The model under review builds one solid part; all positions refer to its coordinate system, in mm. A direction names the side the tool comes from. Round coordinates to 2 decimals unless told otherwise and drop trailing zeros. Order: outer loops, then holes, each group sorted by start corner. A loop starts at its lowest first (then second) coordinate and runs counter-clockwise, first axis right, second up. Notation, with made-up numbers: M -12.5,62 L 32.5,62 A13 ccw 32.5,87 Z; hole C 79,-25 d4. An arc over 180 degrees is marked long. Use a Markdown table: item, result. Add a question column.
1. Insertion check: P1, Ø12, axis at x = 7, z = 6, coming from the +Y side; P2, Ø8, axis at x = 9.5, y = 94.5, coming from the -Z side; P3, Ø5, axis at y = 84.5, z = -6.5, coming from the +X side; P4, Ø4, axis at x = 5.5, z = -13, coming from the -Y side. Each pin has a flat end and moves straight along its axis. Give the tip position at first contact, or say it passes through.
2. Consider section B-B on z = 15. State the section outline as (x, y) points, then the cut area to 3 significant figures.
3. Consider section A-A on x = -10. State the section outline as (y, z) points, then the cut area to 3 significant figures.
4. For faces 1 (the flat face through (-18.5, 148, 0)), 2 (the flat face through (0, 5, -18.3)), 3 (the flat face through (-4, 6.5, 4)), 4 (the flat face through (-1.9, 151, 0)), list the 3-axis set-ups (+Z, -Z, +X, -X, +Y, -Y) from which the entire face can be reached by the end or side of a thin tool; tool diameter is ignored.
5. To check wall thickness, follow probe 1 along Y at (x, z) = (-17, 1); probe 2 along Z at (x, y) = (1, 22.5); probe 3 along X at (y, z) = (7.5, 3). State the ranges of each line that lie inside material, in increasing order.
6. The part is to be moulded in two halves that separate along Y. For faces 5 (the cylindrical face through (0, 13.7, -2.8)), 6 (the flat face through (3, 153, 0)), 7 (the flat face through (0, 10, -18.3)), 8 (the cylindrical face through (-4.88, 7.49, -1.08)), say which applies: +Y half, -Y half, draft (parallel to the pull), parting line (faces both ways), or undercut.
7. Consider section C-C on y = 48. State the section outline as (x, z) points, then the cut area to 3 significant figures.
from build123d import *

# Parameters (mm, degrees)
BOSS_EXTRUDE1_DEPTH     = 6.5
SKETCH2_R               = 20
BOSS_EXTRUDE2_DEPTH     = 2.5
CUT_EXTRUDE1_DEPTH      = 8
SKETCH4_W               = 3
SKETCH4_H               = 3
CUT_EXTRUDE2_DEPTH      = 10
SKETCH5_R               = 5
BOSS_EXTRUDE3_DEPTH     = 140
CUT_EXTRUDE3_DEPTH      = 10
MIRROR5_COPY_1_SKETCH_R = 20
MIRROR5_COPY_1_DEPTH    = 2.5
MIRROR5_COPY_2_SKETCH_W = 3
MIRROR5_COPY_2_SKETCH_H = 3
MIRROR5_COPY_2_DEPTH    = 10


with BuildPart() as part:
    # Sketch1 → Boss-Extrude1 (new body)
    with BuildSketch(Plane(origin=(0, 0, 0), x_dir=(1, 0, 0), z_dir=(0, 1, 0))):
        with BuildLine():
            ThreePointArc((-1.9, -2.05669638), (-2.8, 0), (-1.9, 2.05669638))
            Line((-1.9, 2.05669638), (-1.9, 5.532856405))
            ThreePointArc((-1.9, 5.532856405), (-5.85, 0), (-1.9, -5.532856405))
            Line((-1.9, -5.532856405), (-1.9, -2.05669638))
        make_face()
        with BuildLine():
            ThreePointArc((-1.9, 2.05669638), (0, 2.8), (1.9, 2.05669638))
            Line((1.9, 2.05669638), (1.9, 5.532856405))
            ThreePointArc((1.9, 5.532856405), (0, 5.85), (-1.9, 5.532856405))
            Line((-1.9, 5.532856405), (-1.9, 2.05669638))
        make_face()
        with BuildLine():
            Line((1.9, 5.532856405), (1.9, 2.05669638))
            ThreePointArc((1.9, 2.05669638), (2.565151068, 1.122497216), (2.8, 0))
            ThreePointArc((2.8, 0), (2.565151068, -1.122497216), (1.9, -2.05669638))
            Line((1.9, -2.05669638), (1.9, -5.532856405))
            ThreePointArc((1.9, -5.532856405), (4.761171074, -3.399080758), (5.85, 0))
            ThreePointArc((5.85, 0), (4.761171074, 3.399080758), (1.9, 5.532856405))
        make_face()
        with BuildLine():
            Line((1.9, -5.532856405), (1.9, -2.05669638))
            ThreePointArc((1.9, -2.05669638), (0, -2.8), (-1.9, -2.05669638))
            Line((-1.9, -2.05669638), (-1.9, -5.532856405))
            ThreePointArc((-1.9, -5.532856405), (0, -5.85), (1.9, -5.532856405))
        make_face()
        with BuildLine():
            Line((-1.9, -2.05669638), (-1.9, 2.05669638))
            ThreePointArc((-1.9, 2.05669638), (-2.8, 0), (-1.9, -2.05669638))
        make_face()
        with BuildLine():
            ThreePointArc((2.8, 0), (2.565151068, 1.122497216), (1.9, 2.05669638))
            Line((1.9, 2.05669638), (1.9, -2.05669638))
            ThreePointArc((1.9, -2.05669638), (2.565151068, -1.122497216), (2.8, 0))
        make_face()
    boss_extrude1 = extrude(amount=BOSS_EXTRUDE1_DEPTH)

    # Sketch2 → Boss-Extrude2 (add)
    with BuildSketch(Plane(origin=(0, 6.5, 0), x_dir=(1, 0, 0), z_dir=(0, 1, 0))):
        with Locations(Location((0, 0, 0), (0, 0, 270))):
            Circle(SKETCH2_R)
    boss_extrude2 = extrude(amount=-BOSS_EXTRUDE2_DEPTH)

    # Sketch3 → Cut-Extrude1 (cut)
    with BuildSketch(Plane.XZ.offset(-4)):
        with BuildLine():
            Line((-1.9, 2.05669638), (-1.9, -2.05669638))
            ThreePointArc((-1.9, -2.05669638), (0, -2.8), (1.9, -2.05669638))
            Line((1.9, -2.05669638), (1.9, 2.05669638))
            ThreePointArc((1.9, 2.05669638), (0, 2.8), (-1.9, 2.05669638))
        make_face()
    extrude(amount=-CUT_EXTRUDE1_DEPTH, mode=Mode.SUBTRACT)

    # Sketch4 → Cut-Extrude2 (cut)
    with BuildSketch(Plane(origin=(0, 6.5, 0), x_dir=(1, 0, 0), z_dir=(0, 1, 0))):
        with Locations((0, 19.8)):
            Rectangle(SKETCH4_W, SKETCH4_H)
        with Locations((20, 0)):
            Rectangle(SKETCH4_W, SKETCH4_H)
        with Locations((0, -20)):
            Rectangle(SKETCH4_W, SKETCH4_H)
        with Locations((-20, 0)):
            Rectangle(SKETCH4_W, SKETCH4_H)
    cut_extrude2 = extrude(amount=-CUT_EXTRUDE2_DEPTH, mode=Mode.SUBTRACT)

    # Sketch5 → Boss-Extrude3 (add)
    with BuildSketch(Plane(origin=(0, 6.5, 0), x_dir=(1, 0, 0), z_dir=(0, 1, 0))):
        with Locations(Location((0, 0, 0), (0, 0, 270))):
            Circle(SKETCH5_R)
    extrude(amount=BOSS_EXTRUDE3_DEPTH)

    # Mirror1: Boss-Extrude2, Cut-Extrude2 across plane
    add(boss_extrude2.mirror(Plane.ZX.offset(76.5)))
    add(cut_extrude2.mirror(Plane.ZX.offset(76.5)), mode=Mode.SUBTRACT)

    # Mirror2: Boss-Extrude1 across plane
    add(boss_extrude1.mirror(Plane.ZX.offset(76.5)))

    # Sketch6 → Cut-Extrude3 (cut)
    with BuildSketch(Plane.XZ.offset(-6.5)):
        with BuildLine():
            Line((-1.9, 2.05669638), (-1.9, -2.05669638))
            ThreePointArc((-1.9, -2.05669638), (0, -2.8), (1.9, -2.05669638))
            Line((1.9, -2.05669638), (1.9, 2.05669638))
            ThreePointArc((1.9, 2.05669638), (0, 2.8), (-1.9, 2.05669638))
        make_face()
    extrude(amount=-CUT_EXTRUDE3_DEPTH, mode=Mode.SUBTRACT)

    # Mirror3: Boss-Extrude2, Cut-Extrude2 across plane
    add(boss_extrude2.mirror(Plane.ZX.offset(7.5)))
    add(cut_extrude2.mirror(Plane.ZX.offset(7.5)), mode=Mode.SUBTRACT)

    # Mirror5 copy 1 sketch → Mirror5 copy 1 (add)
    with BuildSketch(Plane(origin=(0, 144.5, 0), x_dir=(1, 0, 0), z_dir=(0, 1, 0))):
        with Locations(Location((0, 0, 0), (0, 0, 270))):
            Circle(MIRROR5_COPY_1_SKETCH_R)
    extrude(amount=-MIRROR5_COPY_1_DEPTH)

    # Mirror5 copy 2 sketch → Mirror5 copy 2 (cut)
    with BuildSketch(Plane(origin=(0, 144.5, 0), x_dir=(1, 0, 0), z_dir=(0, 1, 0))):
        with Locations((0, 19.8)):
            Rectangle(MIRROR5_COPY_2_SKETCH_W, MIRROR5_COPY_2_SKETCH_H)
        with Locations((20, 0)):
            Rectangle(MIRROR5_COPY_2_SKETCH_W, MIRROR5_COPY_2_SKETCH_H)
        with Locations((0, -20)):
            Rectangle(MIRROR5_COPY_2_SKETCH_W, MIRROR5_COPY_2_SKETCH_H)
        with Locations((-20, 0)):
            Rectangle(MIRROR5_COPY_2_SKETCH_W, MIRROR5_COPY_2_SKETCH_H)
    extrude(amount=-MIRROR5_COPY_2_DEPTH, mode=Mode.SUBTRACT)


solid = part.part
Answer block:
| question | item | result |
|---|---|---|
| 1 | P1 | y = 153 |
| 1 | P2 | through |
| 1 | P3 | x = 3 |
| 1 | P4 | y = 4 |
| 2 | outline | M -13.23,4 L 13.23,4 L 13.23,6.5 L -13.23,6.5 Z; M -13.23,8.5 L 13.23,8.5 L 13.23,11 L -13.23,11 Z; M -13.23,142 L 13.23,142 L 13.23,144.5 L -13.23,144.5 Z; M -13.23,146.5 L 13.23,146.5 L 13.23,149 L -13.23,149 Z |
| 2 | area | 265 mm^2 |
| 3 | outline | M 4,-17.32 L 6.5,-17.32 L 6.5,17.32 L 4,17.32 Z; M 8.5,-17.32 L 11,-17.32 L 11,17.32 L 8.5,17.32 Z; M 142,-17.32 L 144.5,-17.32 L 144.5,17.32 L 142,17.32 Z; M 146.5,-17.32 L 149,-17.32 L 149,17.32 L 146.5,17.32 Z |
| 3 | area | 346 mm^2 |
| 4 | face 1 | -X, +Y, -Y |
| 4 | face 2 | -Z, +Y, -Y |
| 4 | face 3 | none |
| 4 | face 4 | +Y |
| 5 | probe 1 | 4 to 6.5, 8.5 to 11, 142 to 144.5, 146.5 to 149 |
| 5 | probe 2 | -4.9 to 4.9 |
| 5 | probe 3 | -4 to 4 |
| 6 | face 5 | undercut |
| 6 | face 6 | +Y half |
| 6 | face 7 | draft |
| 6 | face 8 | undercut |
| 7 | outline | C 0,0 d10 |
| 7 | area | 78.5 mm^2 |
